Check sheet for the modelled part. Datum: model origin and axes. Units: mm. A direction names the side the tool comes from. Round coordinates to 2 decimals unless told otherwise and drop trailing zeros. Order: outer loops, then holes, each group sorted by start corner. A loop starts at its lowest first (then second) coordinate and runs counter-clockwise, first axis right, second up.
Q1. Cross-section at A-A on z = -4.15. Record the cut outline in (x, y), then the cut area to 3 significant figures.
Q2. Scan lines: probe 1 along Z at (x, y) = (11.5, 2.5); probe 2 along X at (y, z) = (8.5, -20); probe 3 along X at (y, z) = (6, -33). Record each from-to range of solid material in increasing order.
Q3. Mould release check, pull along X, two halves, no side actions. Record for faces 5 (the flat face through (0, 3, -20)), 6 (the flat face through (97, 3, -33.75)), 7 (the flat face through (34.8, 15, -20.1)): +X half, -X half, draft (parallel to the pull), parting line (faces both ways), or undercut.
Q4. Cross-section at B-B on y = 2. Give the number of separate pieces and of enclosed holes in the cut face, then the cut area to 3 significant figures.
Q5. Depth check by flat-ended pin: P1, Ø4, axis at x = 55, z = -25, coming from the +Y side; P2, Ø6, axis at x = 23.5, z = -24, coming from the +Y side; P3, Ø2, axis at y = 12, z = -12, coming from the +X side (3 decimals). Enter the tip coordinate at first touch or a pass-through.
Q6. Set-up check for faces 1 (the cylindrical face through (58.507, 9.93, -0.924)), 2 (the flat face through (9, 3, -33.75)), 3 (the flat face through (54, 10, -23)), 4 (the flat face through (8, 7, -20)): record each of +Z, -Z, +X, -X, +Y, -Y from which the full face is reachable in a straight line by a thin tool's end or side.
Q7. Cross-section at D-D on x = 19. Record the cut outline in (y, z).
from build123d import *

# Parameters (mm, degrees)
SKETCH1_W           = 105
SKETCH1_H           = 40
BOSS_EXTRUDE1_DEPTH = 7
SKETCH2_W           = 71
SKETCH2_H           = 40
CUT_EXTRUDE1_DEPTH  = 2
SKETCH4_R           = 20
SKETCH4_R_2         = 17.5
SKETCH4_R_3         = 12.5
BOSS_EXTRUDE3_DEPTH = 10
CUT_EXTRUDE2_START  = -3
SKETCH5_R           = 12.5
CUT_EXTRUDE2_DEPTH  = 3
SKETCH6_R           = 3
SKETCH6_R_2         = 1.75
CUT_EXTRUDE3_DEPTH  = 114
SKETCH7_R           = 4.5
CUT_EXTRUDE4_DEPTH  = 10


with BuildPart() as part:
    # Sketch1 → Boss-Extrude1 (new body)
    with BuildSketch(Plane(origin=(0, 0, 0), x_dir=(1, 0, 0), z_dir=(0, 1, 0))):
        with Locations((52.5, 20)):
            Rectangle(SKETCH1_W, SKETCH1_H)
        with BuildLine():
            Line((4, 37.95), (13, 37.95))
            ThreePointArc((13, 37.95), (15.1, 35.85), (13, 33.75))
            Line((13, 33.75), (4, 33.75))
            ThreePointArc((4, 33.75), (1.9, 35.85), (4, 37.95))
        make_face(mode=Mode.SUBTRACT)
        with BuildLine():
            Line((4, 6.25), (13, 6.25))
            ThreePointArc((13, 6.25), (15.1, 4.15), (13, 2.05))
            Line((13, 2.05), (4, 2.05))
            ThreePointArc((4, 2.05), (1.9, 4.15), (4, 6.25))
        make_face(mode=Mode.SUBTRACT)
        with BuildLine():
            Line((92, 37.95), (101, 37.95))
            ThreePointArc((101, 37.95), (103.1, 35.85), (101, 33.75))
            Line((101, 33.75), (92, 33.75))
            ThreePointArc((92, 33.75), (89.9, 35.85), (92, 37.95))
        make_face(mode=Mode.SUBTRACT)
        with BuildLine():
            Line((92, 6.25), (101, 6.25))
            ThreePointArc((101, 6.25), (103.1, 4.15), (101, 2.05))
            Line((101, 2.05), (92, 2.05))
            ThreePointArc((92, 2.05), (89.9, 4.15), (92, 6.25))
        make_face(mode=Mode.SUBTRACT)
    extrude(amount=BOSS_EXTRUDE1_DEPTH)

    # Sketch2 → Cut-Extrude1 (cut)
    with BuildSketch(Plane(origin=(0, 7, 0), x_dir=(1, 0, 0), z_dir=(0, 1, 0))):
        with Locations((52.5, 20)):
            Rectangle(SKETCH2_W, SKETCH2_H)
    extrude(amount=-CUT_EXTRUDE1_DEPTH, mode=Mode.SUBTRACT)

    # Sketch4 → Boss-Extrude3 (add)
    # profile 1 of 2: a face of its own
    with BuildSketch(Plane(origin=(0, 5, 0), x_dir=(1, 0, 0), z_dir=(0, 1, 0))):
        with Locations(Location((52.5, 20, 0), (0, 0, 270))):
            Circle(SKETCH4_R)
        with Locations(Location((52.5, 20, 0), (0, 0, 270))):
            Circle(SKETCH4_R_2, mode=Mode.SUBTRACT)
    # profile 2 of 2: a face of its own
    with BuildSketch(Plane(origin=(0, 5, 0), x_dir=(1, 0, 0), z_dir=(0, 1, 0))):
        with Locations(Location((52.5, 20, 0), (0, 0, 90))):
            Circle(SKETCH4_R_3)
    extrude(amount=BOSS_EXTRUDE3_DEPTH)

    # Sketch5 → Cut-Extrude2 (cut)
    with BuildSketch(Plane(origin=(0, 15, 0), x_dir=(1, 0, 0), z_dir=(0, 1, 0)).offset(CUT_EXTRUDE2_START)):
        with Locations(Location((52.5, 20, 0), (0, 0, 90))):
            Circle(SKETCH5_R)
    extrude(amount=CUT_EXTRUDE2_DEPTH, mode=Mode.SUBTRACT)

    # Sketch6 → Cut-Extrude3 (cut, through all)
    with BuildSketch(Plane(origin=(0, 12, 0), x_dir=(1, 0, 0), z_dir=(0, 1, 0))):
        with Locations(Location((52.5, 20, 0), (0, 0, 270))):
            Circle(SKETCH6_R)
        with Locations(Location((45.5, 20, 0), (0, 0, 270))):
            Circle(SKETCH6_R_2)
        with Locations(Location((52.5, 27, 0), (0, 0, 270))):
            Circle(SKETCH6_R_2)
        with Locations(Location((59.5, 20, 0), (0, 0, 270))):
            Circle(SKETCH6_R_2)
        with Locations(Location((52.5, 13, 0), (0, 0, 270))):
            Circle(SKETCH6_R_2)
    extrude(amount=-CUT_EXTRUDE3_DEPTH, mode=Mode.SUBTRACT)

    # Sketch7 → Cut-Extrude4 (cut)
    with BuildSketch(Plane.XZ):
        with Locations(Location((52.5, -20, 0), (0, 0, 270))):
            Circle(SKETCH7_R)
    extrude(amount=-CUT_EXTRUDE4_DEPTH, mode=Mode.SUBTRACT)


solid = part.part
Results found:
1. outline: (0, 0) - (1.9, 0) - (1.9, 7) - (0, 7) - close; (15.1, 0) - (89.9, 0) - (89.9, 7) - (88, 7) - (88, 5) - (64.7, 5) - (64.7, 15) - (59.92, 15) - (59.92, 5) - (45.08, 5) - (45.08, 15) - (40.3, 15) - (40.3, 5) - (17, 5) - (17, 7) - (15.1, 7) - close; (103.1, 0) - (105, 0) - (105, 7) - (103.1, 7) - close
1. area: 504 mm2
2. probe 1: z = -40 to -37.95, -33.75 to -6.25, -2.05 to 0
2. probe 2: x = 32.5 to 35, 40 to 43.75, 47.25 to 48, 57 to 57.75, 61.25 to 65, 70 to 72.5
2. probe 3: x = 0 to 17, 37.3 to 40.78, 64.22 to 67.7, 88 to 105
3. face 5: -X half
3. face 6: undercut
3. face 7: draft
4. separate pieces: 1
4. enclosed holes: 9
4. area: 3,890 mm2
5. P1: stops at y = 12
5. P2: stops at y = 5
5. P3: stops at x = 71.235
6. face 1: +Y
6. face 2: +Y, -Y
6. face 3: -Y
6. face 4: +Z, -Z, -X, +Y
7. outline: (0, -40) - (5, -40) - (5, 0) - (0, 0) - close
